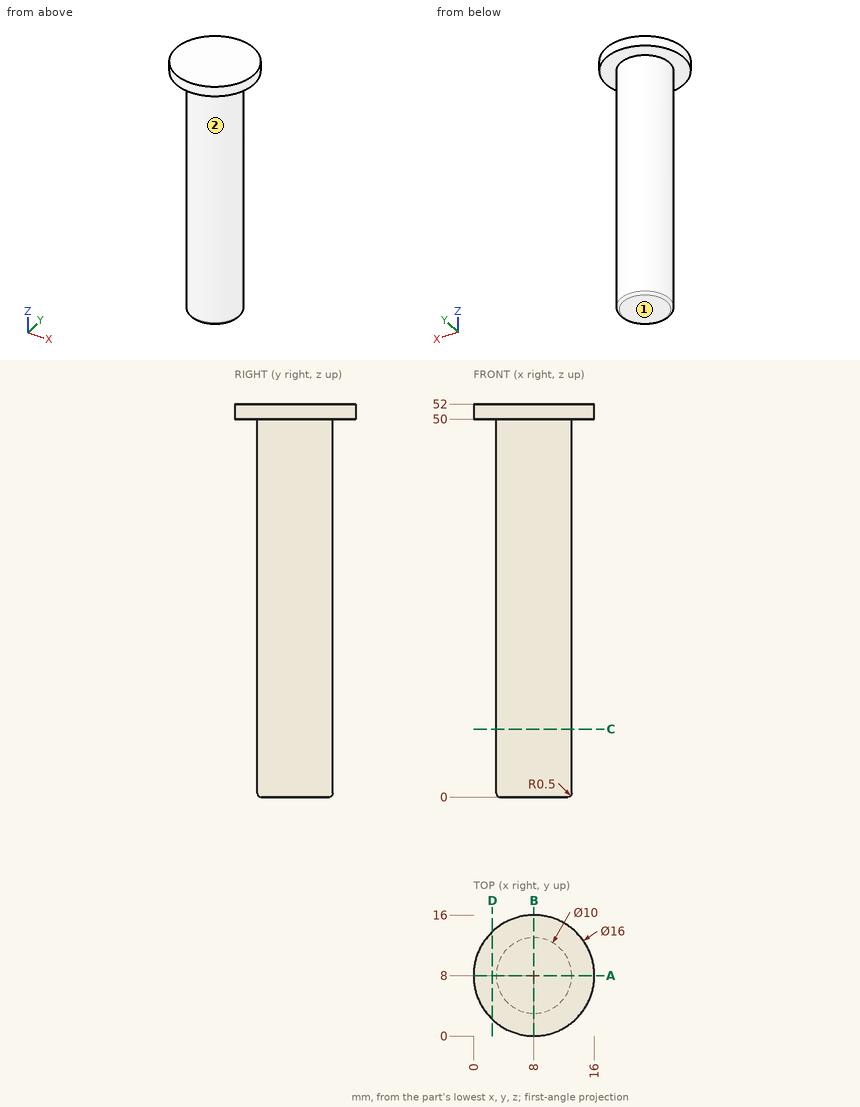
Input: dimensioned drawing with shaded views. Units: mm. Origin: part minimum x, y, z. A direction names the side the tool comes from. Give positions to 0.01 mm unless a question says otherwise; leave off trailing zeros. Write each loop counter-clockwise with the first axis right and the second up, starting at its lowest first coordinate (ties: lowest second). Pieces come first, ordered by that corner, then holes. Notation, with made-up numbers: (71, 49) -> (77, 49) arc R12 cw to (77, 53) -> close; hole circle Ø9 at (-32, 23.25). An arc over 180 degrees is marked (long way). Return JSON: item names as keys, results as strings. Group by question number.
1. Section D-D, the plane x = 2.5. Output: boundary loops of the cut face in (y, z).
2. Material intervals for line 1 (Y direction, x = 7.75, z = 7.5); line 2 (Z direction, x = 8.5, y = 15.25); line 3 (Y direction, x = 6.5, z = 11), sorted ascending. Write a range as from..to.
3. Section C-C, the plane z = 9. Output: boundary loops of the cut face in (x, y), then the cut area to 3 significant figures.
4. Access query for the marked faces 1 and 2. Directions: +Z, -Z, +X, -X, +Y, -Y. A direction counts if a zero-diameter tool reaches every point of the face in a straight line with its end or side. Return the directions, or none.
5. Section A-A, the plane y = 8. Output: boundary loops of the cut face in (x, z).
6. Pin query (flat end, axial travel): pin 1 Ø1 at (x, z) = (12.5, 30.5) entering from -Y; pin 2 Ø6 at (y, z) = (3.5, 35.5) entering from -X; pin 3 Ø3 at (y, z) = (11.5, 40) entering from +X. Return the tip coordinate at first contact, or that it passes through.
Determined:
{
 "1": {"outline": "(2.19, 50) -> (13.81, 50) -> (13.81, 52) -> (2.19, 52) -> close"},
 "2": {"line 1": "y = 3.01..12.99", "line 2": "z = 50..52", "line 3": "y = 3.23..12.77"},
 "3": {"outline": "circle Ø10 at (8, 8)", "area": "78.5 mm2"},
 "4": {"face 1": "-Z, +X, -X, +Y, -Y", "face 2": "-Z"},
 "5": {"outline": "(0, 50) -> (3, 50) -> (3, 0.5) arc R0.5 ccw to (3.5, 0) -> (12.5, 0) arc R0.5 ccw to (13, 0.5) -> (13, 50) -> (16, 50) -> (16, 52) -> (0, 52) -> close"},
 "6": {"pin 1": "stops at y = 5", "pin 2": "stops at x = 3.23", "pin 3": "stops at x = 12.58"}
}
